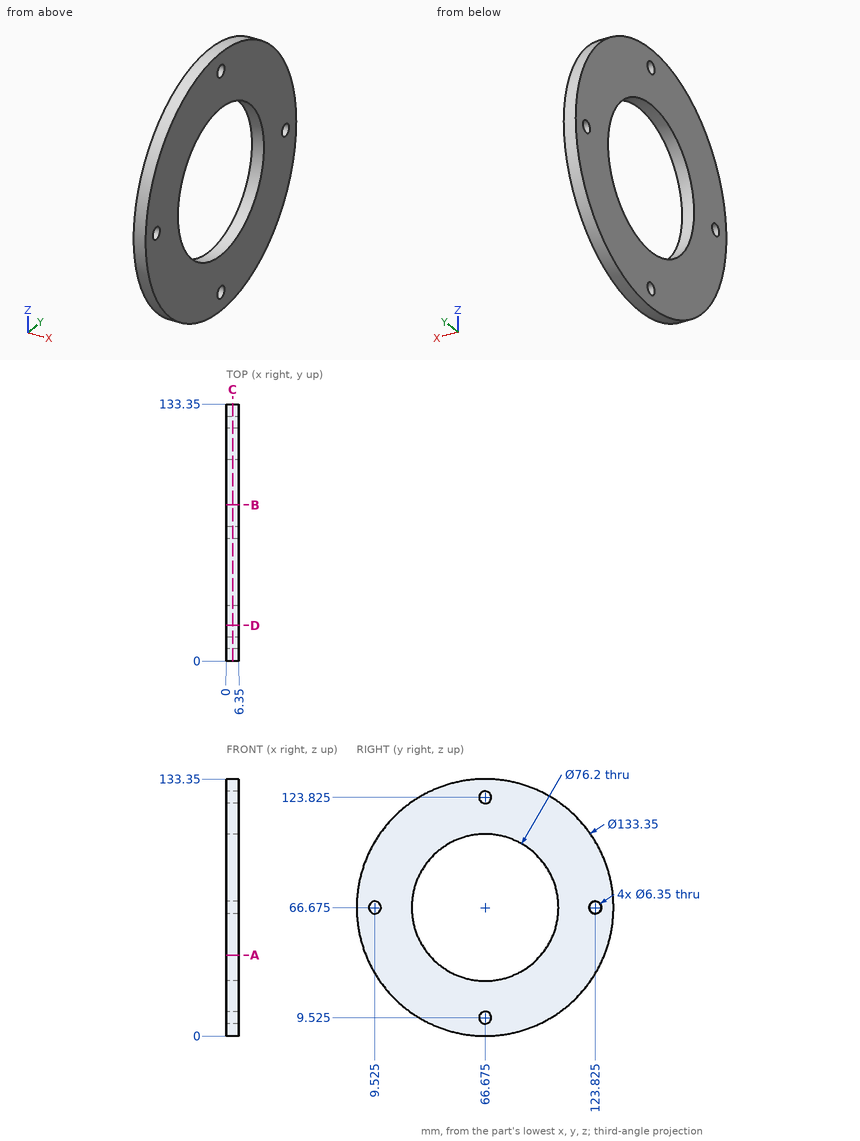
The figure shows three views and two pictorial views of one solid part (mm, origin at its lowest corner). Answer the questions. Give positions to 0.01 mm unless a question says otherwise; leave off trailing zeros. Loops run counter-clockwise (first coordinate to the right, second up) from the corner with the lowest first, then second, coordinate; pieces in that order, holes last. Notation, with made-up numbers: (3, 41) -> (10, 41) arc R27 ccw to (10, 60) -> close; hole circle Ø7 at (28, 67). An arc over 180 degrees is marked (long way). Use a Markdown table: item, result. Add a question column.
1. Section B-B on y = 81 is taken. Determine the outline of the cut face in (x, z).
2. Section D-D on y = 18.5 is taken. Determine the outline of the cut face in (x, z), and give its area (3 significant figures).
3. Section C-C on x = 3.25 is taken. Determine the outline of the cut face in (y, z) (3 decimals), and give its area (3 significant figures).
4. Find the intervals of material crossed by probe 1 along Z at (x, y) = (3.25, 100); probe 2 along Y at (x, z) = (4, 76); probe 3 along Y at (x, z) = (5, 93), in increasing order.
5. Section A-A on z = 42 is taken. Determine the outline of the cut face in (x, y), and give its area (3 significant figures).
6. Flat-ended cylindrical pins translate along their axes: pin 1 Ø10 at (y, z) = (123.825, 66.675) entering from +X; pin 2 Ø3 at (x, z) = (3, 43) entering from -Y; pin 3 Ø3 at (x, y) = (3, 93) entering from -Z; pin 4 Ø4 at (y, z) = (9.525, 66.675) entering from +X. Find the tip coordinate at first contact, or state that the pin passes through.
Results below:
| question | item | result |
|---|---|---|
| 1 | outline | (0, 1.56) -> (6.35, 1.56) -> (6.35, 31.37) -> (0, 31.37) -> close; (0, 101.98) -> (6.35, 101.98) -> (6.35, 131.79) -> (0, 131.79) -> close |
| 2 | outline | (0, 20.58) -> (6.35, 20.58) -> (6.35, 112.77) -> (0, 112.77) -> close |
| 2 | area | 585 mm^2 |
| 3 | outline | circle Ø133.35 at (66.675, 66.675); hole circle Ø6.35 at (9.525, 66.675); hole circle Ø76.2 at (66.675, 66.675); hole circle Ø6.35 at (66.675, 9.525); hole circle Ø6.35 at (66.675, 123.825); hole circle Ø6.35 at (123.825, 66.675) |
| 3 | area | 9,280 mm^2 |
| 4 | probe 1 | z = 8.93 to 48.21, 85.14 to 124.42 |
| 4 | probe 2 | y = 0.66 to 29.73, 103.62 to 132.69 |
| 4 | probe 3 | y = 5.42 to 39.13, 94.22 to 127.93 |
| 5 | outline | (0, 4.73) -> (6.35, 4.73) -> (6.35, 37.64) -> (0, 37.64) -> close; (0, 95.71) -> (6.35, 95.71) -> (6.35, 128.62) -> (0, 128.62) -> close |
| 5 | area | 418 mm^2 |
| 6 | pin 1 | stops at x = 6.35 |
| 6 | pin 2 | stops at y = 3.8 |
| 6 | pin 3 | stops at z = 4.79 |
| 6 | pin 4 | passes through |
